from build123d import *

# Parameters (mm, degrees)
SKETCH2_R               = 11.96975
SKETCH2_R_2             = 2.44475
BOSS_EXTRUDE1_DEPTH     = 5.588
CUT_EXTRUDE1_DEPTH      = 2.54
CUT_EXTRUDE1_DEPTH_BACK = 15
SKETCH3_R               = 1.35255
BOSS_EXTRUDE2_START     = 18.588
SKETCH4_R               = 11.96975
BOSS_EXTRUDE2_DEPTH     = 18.588
SKETCH5_R               = 2.563495
CUT_EXTRUDE3_DEPTH      = 12
CUT_EXTRUDE4_DEPTH      = 1.27
CUT_EXTRUDE4_DEPTH_BACK = 12.446
SKETCH6_R               = 1.35255
SKETCH10_R              = 2.0193
CUT_EXTRUDE6_DEPTH      = 11.43


with BuildPart() as part:
    # Sketch2 → Boss-Extrude1 (new body)
    with BuildSketch(Plane(origin=(0, 0, 0), x_dir=(1, 0, 0), z_dir=(0, 1, 0))):
        with Locations(Location((0, 0, 0), (0, 0, 270))):
            Circle(SKETCH2_R)
        with Locations(Location((0, 0, 0), (0, 0, 270))):
            Circle(SKETCH2_R_2, mode=Mode.SUBTRACT)
    extrude(amount=BOSS_EXTRUDE1_DEPTH)

    # Sketch3 → Cut-Extrude1 (cut, two sides: drawn at the far end of the back side and taken through both)
    with BuildSketch(Plane(origin=(-1.039168295, 0, 2.212901222), x_dir=(-0.9051646270437873, 0, -0.425061169655241), z_dir=(0.425061169655241, 0, -0.9051646270437873)).offset(-CUT_EXTRUDE1_DEPTH_BACK)):
        with Locations(Location((0, 3.302, 0), (0, 0, 180))):
            Circle(SKETCH3_R)
    extrude(amount=CUT_EXTRUDE1_DEPTH + CUT_EXTRUDE1_DEPTH_BACK, mode=Mode.SUBTRACT)

    # Sketch4 → Boss-Extrude2 (add)
    with BuildSketch(Plane(origin=(0, 0, 0), x_dir=(-1, 0, 0), z_dir=(0, -1, 0)).offset(BOSS_EXTRUDE2_START)):
        with Locations(Location((0, 0, 0), (0, 0, 90))):
            Circle(SKETCH4_R)
    extrude(amount=-BOSS_EXTRUDE2_DEPTH)

    # Sketch5 → Cut-Extrude3 (cut)
    with BuildSketch(Plane(origin=(0, -18.588, 0), x_dir=(-1, 0, 0), z_dir=(0, -1, 0))):
        with Locations(Location((0, 0, 0), (0, 0, 90))):
            Circle(SKETCH5_R)
    extrude(amount=-CUT_EXTRUDE3_DEPTH, mode=Mode.SUBTRACT)

    # Sketch6 → Cut-Extrude4 (cut, two sides: drawn at the far end of the back side and taken through both)
    with BuildSketch(Plane(origin=(-1.039168295, 0, 2.212901222), x_dir=(-0.9051646270437873, 0, -0.425061169655241), z_dir=(0.425061169655241, 0, -0.9051646270437873)).offset(-CUT_EXTRUDE4_DEPTH_BACK)):
        with Locations(Location((0, -13.588, 0), (0, 0, 180))):
            Circle(SKETCH6_R)
    extrude(amount=CUT_EXTRUDE4_DEPTH + CUT_EXTRUDE4_DEPTH_BACK, mode=Mode.SUBTRACT)

    # Sketch10 → Cut-Extrude6 (cut)
    with BuildSketch(Plane(origin=(-4.063543521, 0, -11.258886673), x_dir=(0, -1, 0), z_dir=(-0.3394844103905428, 0, -0.9406116813551624))):
        with Locations(Location((13.762, 0, 0), (0, 0, 90))):
            Circle(SKETCH10_R)
        with Locations(Location((-2.794, 0, 0), (0, 0, 90))):
            Circle(SKETCH10_R)
    extrude(amount=-CUT_EXTRUDE6_DEPTH, mode=Mode.SUBTRACT)


solid = part.part
Model file for the job. Use its own axes, mm. A direction names the side the tool comes from. Give positions to 0.01 mm unless a question says otherwise; leave off trailing zeros. Order: outer loops, then holes, each group sorted by start corner. A loop starts at its lowest first (then second) coordinate and runs counter-clockwise, first axis right, second up. Notation, with made-up numbers: (12.5, 81) - (55.5, 81) arc R31 ccw to (55.5, 114) - close; hole circle Ø1 at (-14, 66). An arc over 180 degrees is marked (long way). One line per item, written item: value.
Item 1: Slice it at B-B (y = -7.5). List the corners of the cut face in (x, z), then the cut area to 3 significant figures.
Response values:
outline: circle Ø23.94 at (0, 0); hole circle Ø5.13 at (0, 0)
area: 429 mm2
Item 2: Slice it at D-D (z = 8.75). Give the number of separate pieces and of enclosed holes in the cut face, then the cut area to 3 significant figures.
Response values:
separate pieces: 1
enclosed holes: 2
area: 382 mm2
Item 3: Tool access for faces 1 (the flat face through (0, -6.588, 0)), 2 (the cylindrical face through (-3.2, -14.93, 6.39)), 3 (the flat face through (0, 0, 0)): list every direction of +Z, -Z, +X, -X, +Y, -Y with a clear straight run to the whole face (end or side of a thin tool).
Response values:
face 1: -Y
face 2: none
face 3: +Y
Item 4: Wall check: line 1 (X direction, y = -9.25, z = 0); line 2 (X direction, y = 1.5, z = 0). Give the ranges that are in metal, low to high.
Response values:
line 1: -11.97 to -2.56, 2.56 to 11.97
line 2: -11.97 to -2.44, 2.44 to 11.97
Item 5: Slice it at C-C (x = 8.5). List the corners of the cut face in (y, z), then the cut area to 3 significant figures.
Response values:
outline: (-18.59, -8.43) - (5.59, -8.43) - (5.59, 8.43) - (-18.59, 8.43) - close
area: 407 mm2
Item 6: Two-plate mould, pull along Z, no slides. Class faces 4 (the cylindrical face through (-0.43, -13.67, -7.13)), 5 (the cylindrical face through (-2.44, 4.5, 6.67)), 6 (the flat face through (3, 5.588, 0)), 7 (the cylindrical face through (11.944, -6.669, -0.789)): released by +Z, released by -Z, zero draft, split by the parting line, or undercut.
Response values:
face 4: undercut
face 5: undercut
face 6: zero draft
face 7: split by the parting line
Item 7: Slice it at A-A (z = 0). List the corners of the cut face in (x, y), then the cut area to 3 significant figures.
Response values:
outline: (-11.97, -18.59) - (-2.56, -18.59) - (-2.56, -6.59) - (2.56, -6.59) - (2.56, -18.59) - (11.97, -18.59) - (11.97, 5.59) - (2.44, 5.59) - (2.44, 0) - (-2.44, 0) - (-2.44, 5.59) - (-11.97, 5.59) - close
area: 490 mm2
Item 8: Pin check, flat tips, straight feed: pin 1 Ø2 at (x, y) = (-2.5, -7) entering from -Z; pin 2 Ø1.5 at (y, z) = (-5, 7) entering from -X; pin 3 Ø2.5 at (x, z) = (0.5, 0) entering from -Y. Stop position of each tip, or through.
Response values:
pin 1: z = -11.88
pin 2: x = -10.21
pin 3: y = -6.59
